Here's how the part is built. I have some questions about the finished solid (model axes, mm). Face numbers are marked on the shaded views. A direction names the side the tool comes from. Coordinates: 2 decimals unless noted, no trailing zeros. Write each loop counter-clockwise with the first axis right and the second up, starting at its lowest first coordinate (ties: lowest second). Pieces come first, ordered by that corner, then holes. Notation, with made-up numbers: M -15.5,3.5 L -0.5,3.5 A20 cw -0.5,38.5 Z; hole C 42,89 d10. An arc over 180 degrees is marked long. Use one line per item in the form item = value. Start each with the question number.
1. I'm going to push flat-ended pins straight in: pin 1 Ø0.8 at (x, z) = (-0.5, -5.5) entering from +Y; pin 2 Ø1.5 at (y, z) = (-2, 6) entering from -X; pin 3 Ø4 at (x, z) = (0, 71.5) entering from +Y (3 decimals); pin 4 Ø1.4 at (x, y) = (0, 0) entering from -Z (3 decimals). Where does each tip first touch, or does it pass through?
2. Please list where these lines run through material, in increasing order: line 1 along X through (y, z) = (-1.75, 26); line 2 along Z through (x, y) = (2.25, 3.5). Write a range as [from, to].
3. I want a section at B-B, the plane z = 21.5. List the corners of the cut face in (x, y) for me (3 decimals).
4. On a 3-axis mill with a long thin cutter (end or side, diameter ignored), from which of +Z, -Z, +X, -X, +Y, -Y can I reach the whole of each face in a straight line? I mean the marked faces 1 and 2. Say none if no direction works.
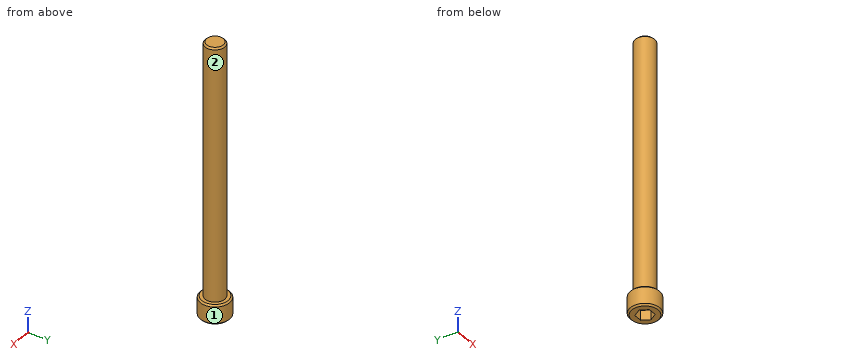
Autodesk Inventor part; units mm, degrees
ref_plane "YZ Plane" through (0, 0, 0) normal (1, 0, 0) x (0, 1, 0)
ref_plane "XZ Plane" through (0, 0, 0) normal (0, 1, 0) x (-1, 0, 0)
ref_plane "XY Plane" through (0, 0, 0) normal (0, 0, 1) x (1, 0, 0)
sketch "Sketch1" plane through (0, 0, 0) normal (0, 0, 1) x (1, 0, 0)
  circle A0 centre (0, 0) radius 3.175
  dimension "d0" = 6.35
extrude "Extrusion1" add sketch "Sketch1" along normal blind 82.55
sketch "Sketch2" plane through (0, 0, 0) normal (0, 0, -1) x (-1, 0, 0)
  circle A0 centre (0, 0) radius 3.175
  circle A1 centre (0, 0) radius 4.7625
  dimension "d3" = 9.525
extrude "Extrusion2" add sketch "Sketch2" along normal blind 6.35 contours A0 | A1
sketch "Sketch3" plane through (0, 0, -6.35) normal (0, 0, -1) x (-1, 0, 0)
  circle A0 centre (0, 0) radius 4.7625
  line L0 (-1.3748, 2.3812) -> (1.3748, 2.3813)
  line L1 (1.3748, 2.3813) -> (2.7496, 0)
  line L2 (2.7496, 0) -> (1.3748, -2.3812)
  line L3 (1.3748, -2.3812) -> (-1.3748, -2.3812)
  line L4 (-1.3748, -2.3812) -> (-2.7496, 0)
  line L5 (-2.7496, 0) -> (-1.3748, 2.3812)
  dimension "d6" = 4.7625
extrude "Extrusion3" cut sketch "Sketch3" against normal blind 3.175 contours L0 L1 L2 L3 L4 L5
chamfer "Chamfer1" distance 0.508 angle 45 3 edges at (-3.175, 0, 82.55) (4.7625, 0, 0) (4.7625, 0, -6.35)
thread "Thread1"
properties part number "14-20 x750" material "Steel"
Answer list:
q1.pin_1 = 4.76
q1.pin_2 = -2.92
q1.pin_3 = 3.175
q1.pin_4 = -3.175
q2.line_1 = [-2.65, 2.65]
q2.line_2 = [-6.35, 0]
q3.outline = C 0,0 d6.35
q4.face_1 = +Z, -Z
q4.face_2 = +Z
